Design review of the part built by this model. Coordinates are the model's own, in mm. A direction names the side the tool comes from. Round coordinates to 2 decimals unless told otherwise and drop trailing zeros. Order: outer loops, then holes, each group sorted by start corner. A loop starts at its lowest first (then second) coordinate and runs counter-clockwise, first axis right, second up. Notation, with made-up numbers: M -23,20.5 L 25,20.5 A17 cw 25,27.5 Z; hole C -39,2.5 d9. An arc over 180 degrees is marked long. Write each question's results on one line, items separated by ' | '. Start each with the question number.
Item 1: Machinability: for faces 1 (the flat face through (36.1, 8, 88)), 2 (the flat face through (38.8, 8, 2)), 3 (the flat face through (37, 8, 1)), which of the approach directions +Z, -Z, +X, -X, +Y, -Y give a long, thin tool a straight path to every point of the face, cutting with its end or side? Answer none if there is none.
Item 2: Clearance check with flat-ended pins moving along their axes: pin 1 (3 mm diameter, centred on x = 2, y = 7, fed in from -Z); pin 2 (6 mm diameter, centred on x = 16, z = 48, fed in from +Y); pin 3 (0.8 mm diameter, centred on y = 6.5, z = 2, fed in from +X). State where each tip first meets the part, or that it passes through.
Item 3: Wall thickness on line 1 (X direction, y = 1.1, z = 45); line 2 (Y direction, x = 16.5, z = 45); line 3 (Z direction, x = 56.5, y = 1): over which ranges is each line inside the solid? List them lowest first. Write a range as [from, to].
Item 4: Take a section at C-C, the plane x = 53. Write out the cut boundary in (y, z), plus the area to 3 significant figures.
Item 5: Take a section at B-B, the plane z = 45. Write out the cut boundary in (x, y), plus the area to 3 significant figures.
Item 6: Take a section at A-A, the plane x = 45. Write out the cut boundary in (y, z), plus the area to 3 significant figures.
Item 7: Take a section at D-D, the plane z = 80. Write out the cut boundary in (x, y), plus the area to 3 significant figures.
```python
from build123d import *

# Parameters (mm, degrees)
SKETCH1_W           = 75
SKETCH1_H           = 90
BOSS_EXTRUDE1_DEPTH = 3
SKETCH2_W           = 2.7
SKETCH2_H           = 2.7
BOSS_EXTRUDE2_DEPTH = 10
SKETCH3_R           = 26
CUT_EXTRUDE1_DEPTH  = 3


with BuildPart() as part:
    # Sketch1 → Boss-Extrude1 (new body)
    with BuildSketch(Plane(origin=(0, 0, 0), x_dir=(1, 0, 0), z_dir=(0, 1, 0))):
        with Locations((37.5, -45)):
            Rectangle(SKETCH1_W, SKETCH1_H)
    extrude(amount=BOSS_EXTRUDE1_DEPTH)

    # Sketch2 → Boss-Extrude2 (add)
    with BuildSketch(Plane(origin=(0, 3, 0), x_dir=(1, 0, 0), z_dir=(0, 1, 0))):
        with Locations((37.45, -2.35)):
            Rectangle(SKETCH2_W, SKETCH2_H)
        with Locations((2.35, -45)):
            Rectangle(SKETCH2_W, SKETCH2_H)
        with Locations((37.45, -87.65)):
            Rectangle(SKETCH2_W, SKETCH2_H)
    extrude(amount=BOSS_EXTRUDE2_DEPTH)

    # Sketch3 → Cut-Extrude1 (cut)
    with BuildSketch(Plane(origin=(0, 3, 0), x_dir=(1, 0, 0), z_dir=(0, 1, 0))):
        with Locations(Location((45, -45, 0), (0, 0, 270))):
            Circle(SKETCH3_R)
    extrude(amount=-CUT_EXTRUDE1_DEPTH, mode=Mode.SUBTRACT)


solid = part.part
```
Results list:
1) face 1: +Z, -Z, -X, +Y | face 2: +Z, -Z, +X, +Y | face 3: -Z, +X, -X, +Y
2) pin 1: z = 43.65 | pin 2: y = 3 | pin 3: x = 38.8
3) line 1: [0, 19], [71, 75] | line 2: [0, 3] | line 3: [0, 21.68], [68.32, 90]
4) outline: M 0,0 L 3,0 L 3,20.26 L 0,20.26 Z; M 0,69.74 L 3,69.74 L 3,90 L 0,90 Z | area: 122 mm²
5) outline: M 0,0 L 19,0 L 19,3 L 3.7,3 L 3.7,13 L 1,13 L 1,3 L 0,3 Z; M 71,0 L 75,0 L 75,3 L 71,3 Z | area: 96.0 mm²
6) outline: M 0,0 L 3,0 L 3,19 L 0,19 Z; M 0,71 L 3,71 L 3,90 L 0,90 Z | area: 114 mm²
7) outline: M 0,0 L 75,0 L 75,3 L 0,3 Z | area: 225 mm²
